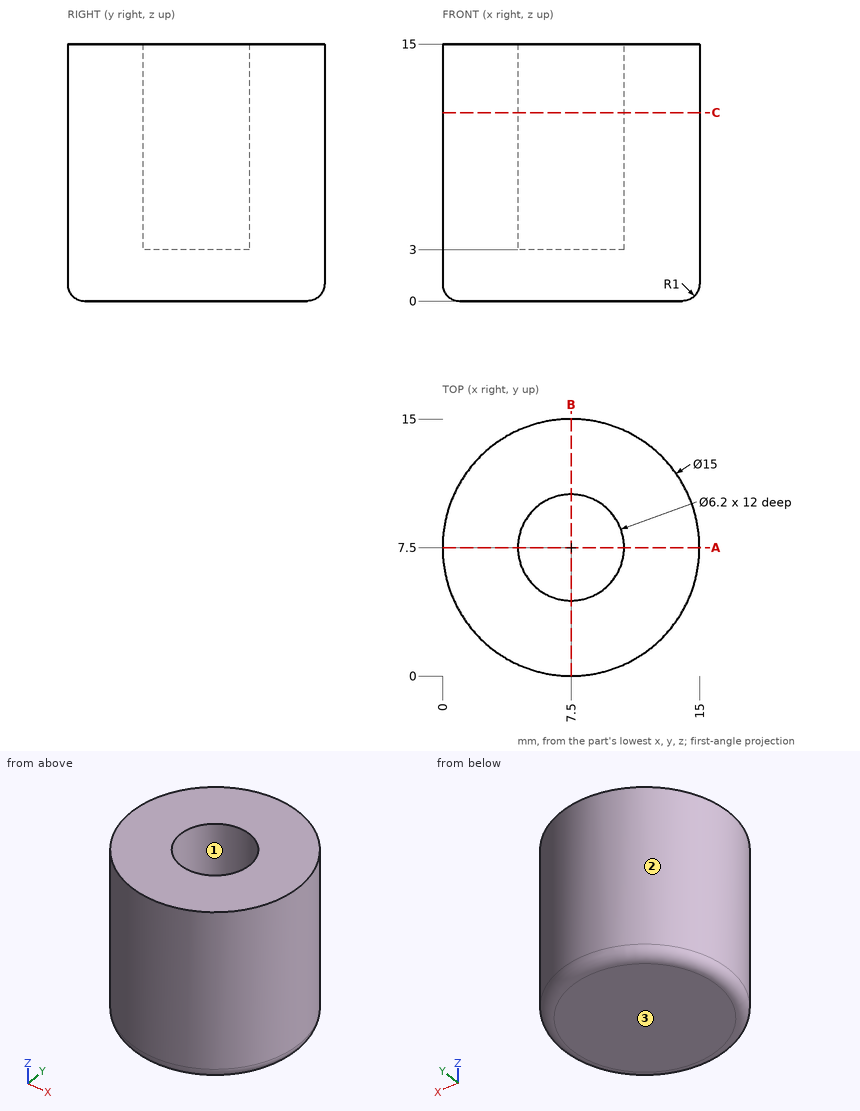
The drawing under review shows one solid part. Ordinate dimensions are in mm from its lowest x, y, z. Coordinates: 2 decimals unless noted, no trailing zeros. Order: outer loops, then holes, each group sorted by start corner. A loop starts at its lowest first (then second) coordinate and runs counter-clockwise, first axis right, second up. Notation, with made-up numbers: (28, 86) - (81, 86) arc R24 cw to (81, 104) - close; hole circle Ø9 at (20, 5). An arc over 180 degrees is marked (long way). Put each result on its own line as item: value.
1) The part is to be moulded in two halves that separate along X. For the marked faces 1, 2 and 3, say which applies: released by +X, released by -X, zero draft, split by the parting line, or undercut.
Response values:
face 1: undercut
face 2: split by the parting line
face 3: zero draft
2) Take a section at A-A, the plane y = 7.5. Give the boundary of the cut face in (x, z).
Response values:
outline: (0, 1) arc R1 ccw to (1, 0) - (14, 0) arc R1 ccw to (15, 1) - (15, 15) - (10.6, 15) - (10.6, 3) - (4.4, 3) - (4.4, 15) - (0, 15) - close
3) Insertion check: P1, Ø5, axis at x = 12.5, z = 7.5, coming from the -Y side; P2, Ø2, axis at x = 3.5, z = 10.5, coming from the -Y side. Each pin has a flat end and moves straight along its axis. Give the tip position at first contact, or say it passes through.
Response values:
P1: stops at y = 0.43
P2: stops at y = 0.63
4) Take a section at C-C, the plane z = 11. Give the boundary of the cut face in (x, y), and give its area (3 significant figures).
Response values:
outline: circle Ø15 at (7.5, 7.5); hole circle Ø6.2 at (7.5, 7.5)
area: 147 mm²
5) Wall thickness on L1, parallel to Y at x = 7.5, z = 11; L2, parallel to Z at x = 10, y = 6; L3, parallel to X at y = 8, z = 8.5: over which ranges is each line inside the solid? List them lowest first. Write a range as from..to.
Response values:
L1: y = 0..4.4, 10.6..15
L2: z = 0..3
L3: x = 0.02..4.44, 10.56..14.98
